```python
from build123d import *

# Parameters (mm, degrees)
SKETCH1_R           = 152.5
SKETCH1_R_2         = 10
BOSS_EXTRUDE1_DEPTH = 10
SKETCH2_R           = 20
SKETCH2_R_2         = 10
BOSS_EXTRUDE2_DEPTH = 30
SKETCH3_R           = 2
CUT_EXTRUDE1_DEPTH  = 60


with BuildPart() as part:
    # Sketch1 → Boss-Extrude1 (new body)
    with BuildSketch(Plane.XY):
        Circle(SKETCH1_R)
        Circle(SKETCH1_R_2, mode=Mode.SUBTRACT)
    extrude(amount=BOSS_EXTRUDE1_DEPTH)

    # Sketch2 → Boss-Extrude2 (add)
    with BuildSketch(Plane.XY.offset(10)):
        Circle(SKETCH2_R)
        Circle(SKETCH2_R_2, mode=Mode.SUBTRACT)
    extrude(amount=BOSS_EXTRUDE2_DEPTH)

    # Sketch3 → Cut-Extrude1 (cut)
    with BuildSketch(Plane(origin=(0, 0, 0), x_dir=(1, 0, 0), z_dir=(0, 1, 0))):
        with Locations(Location((0, -31.638618724, 0), (0, 0, 270))):  # turned: the seam where the file's is
            Circle(SKETCH3_R)
    extrude(amount=-CUT_EXTRUDE1_DEPTH, mode=Mode.SUBTRACT)


solid = part.part
```
CAD build for the part. Positions are in the model's coordinates, mm. A direction names the side the tool comes from. Round coordinates to 2 decimals unless told otherwise and drop trailing zeros. Write each loop counter-clockwise with the first axis right and the second up, starting at its lowest first coordinate (ties: lowest second). Pieces come first, ordered by that corner, then holes.
Item 1: Mould opens along Y. For faces 1 (the cylindrical face through (-152.353, 6.705, 4.93)), 2 (the cylindrical face through (-2.17, -9.76, 19.72)), 3 (the flat face through (-5, 9, 40)) say: released by +Y, released by -Y, zero draft, split by the parting line, or undercut.
Filled in:
face 1: split by the parting line
face 2: undercut
face 3: zero draft
Item 2: Drop flat-ended pins along their axis: pin 1 Ø1 at (x, y) = (52.5, 37) entering from -Z; pin 2 Ø4 at (x, z) = (-105.5, 6.5) entering from +Y; pin 3 Ø3 at (y, z) = (118, 5.5) entering from +X; pin 4 Ø12 at (y, z) = (47.5, 17.5) entering from -X. Give the stop position or say it passes through.
Filled in:
pin 1: stops at z = 0
pin 2: stops at y = 112
pin 3: stops at x = 98.41
pin 4: passes through
Item 3: Band-saw the part on C-C on x = -32. Write the cut outline in (y, z), then the cut area to 3 significant figures.
Filled in:
outline: (-149.1, 0) - (149.1, 0) - (149.1, 10) - (-149.1, 10) - close
area: 2,980 mm2
Item 4: Tool access for faces 4 (the cylindrical face through (-4.336, -19.524, 24.79)), 5 (the flat face through (32, 2, 0)): list every direction of +Z, -Z, +X, -X, +Y, -Y with a clear straight run to the whole face (end or side of a thin tool).
Filled in:
face 4: +Z
face 5: -Z, +X, -X, +Y, -Y
Item 5: Band-saw the part on A-A on y = 0. Write the cut outline in (x, z), then the cut area to 3 significant figures.
Filled in:
outline: (-152.5, 0) - (-10, 0) - (-10, 40) - (-20, 40) - (-20, 10) - (-152.5, 10) - close; (10, 0) - (152.5, 0) - (152.5, 10) - (20, 10) - (20, 40) - (10, 40) - close
area: 3,450 mm2
Item 6: Band-saw the part on D-D on y = -37.5. Write the cut outline in (x, z), then the cut area to 3 significant figures.
Filled in:
outline: (-147.82, 0) - (147.82, 0) - (147.82, 10) - (-147.82, 10) - close
area: 2,960 mm2
Item 7: Band-saw the part on B-B on z = 4. Write the cut outline in (x, y).
Filled in:
outline: circle Ø305 at (0, 0); hole circle Ø20 at (0, 0)
Item 8: Drill centre lines: L1, parallel to Z at x = 0, y = -12.75; L2, parallel to Y at x = 0, z = 16.5; L3, parallel to Z at x = -56, y = -109. Where is each one in solid material? Low to high.
Filled in:
L1: z = 0 to 29.64, 33.64 to 40
L2: y = -20 to -10, 10 to 20
L3: z = 0 to 10
